Could you check a few things on this model? Use its own coordinates, in mm. Give positions to 0.01 mm unless a question says otherwise; leave off trailing zeros. Write each loop counter-clockwise with the first axis right and the second up, starting at its lowest first coordinate (ties: lowest second). Pieces come first, ordered by that corner, then holes. Notation, with made-up numbers: (58.25, -6) - (84.25, -6) arc R30 cw to (84.25, 31) - close; hole circle Ø2 at (58, 40). An arc over 180 degrees is marked (long way). Answer in a Markdown table with one row per item.
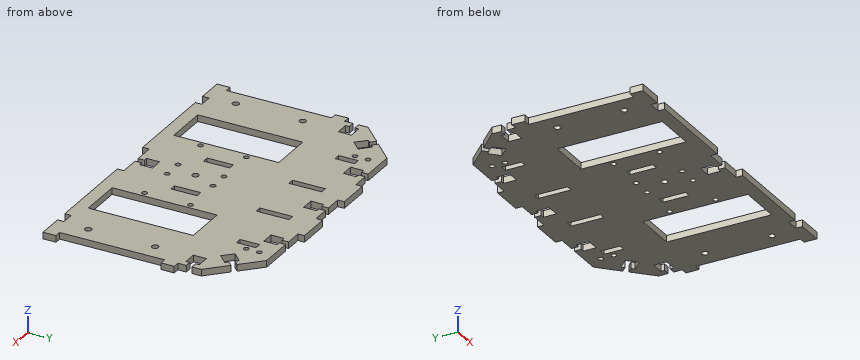
from build123d import *

# Parameters (mm, degrees)
BOSS_EXTRUDE1_DEPTH  = 5
BOSS_EXTRUDE2_DEPTH  = 5
SKETCH3_R            = 2
SKETCH3_R_2          = 2.5
CUT_EXTRUDE4_DEPTH   = 10
SKETCH6_R            = 2.5
CUT_EXTRUDE5_DEPTH   = 10
CUT_EXTRUDE6_DEPTH   = 10
SKETCH9_W            = 35
SKETCH9_H            = 5
SKETCH9_W_2          = 4.2
SKETCH9_W_3          = 10
SKETCH9_H_2          = 10
CUT_EXTRUDE7_DEPTH   = 10
SKETCH10_W           = 30.598870639
SKETCH10_H           = 58.148019952
CUT_EXTRUDE8_DEPTH   = 5
SKETCH11_W           = 30
SKETCH11_H           = 5
CUT_EXTRUDE9_DEPTH   = 5
SKETCH12_W           = 5
SKETCH12_H           = 80
BOSS_EXTRUDE3_DEPTH  = 4.5
SKETCH13_W           = 5
SKETCH13_H           = 80
BOSS_EXTRUDE4_DEPTH  = 4.5
SKETCH14_W           = 5
SKETCH14_H           = 5
BOSS_EXTRUDE5_DEPTH  = 0.1
SKETCH15_W           = 5
SKETCH15_H           = 5
CUT_EXTRUDE10_DEPTH  = 0.1
SKETCH16_W           = 5
SKETCH16_H           = 5
BOSS_EXTRUDE6_DEPTH  = 0.1
SKETCH17_W           = 5
SKETCH17_H           = 5
CUT_EXTRUDE11_DEPTH  = 0.1
SKETCH18_W           = 315.275634843
SKETCH18_H           = 155.272188677
CUT_EXTRUDE12_DEPTH  = 0.1
SKETCH19_W           = 15.4
SKETCH19_H           = 5
CUT_EXTRUDE13_DEPTH  = 0.1
CUT_EXTRUDE14_DEPTH  = 5
SKETCH21_W           = 5
SKETCH21_H           = 4.2
SKETCH21_W_2         = 3.2
SKETCH21_W_3         = 1.8
SKETCH21_H_2         = 1.4
CUT_EXTRUDE15_DEPTH  = 5
SKETCH22_W           = 5
SKETCH22_H           = 25
CUT_EXTRUDE16_DEPTH  = 10
SKETCH23_R           = 2
CUT_EXTRUDE17_DEPTH  = 10
CUT_EXTRUDE18_DEPTH  = 10
SKETCH25_W           = 5
SKETCH25_H           = 5
BOSS_EXTRUDE7_DEPTH  = 5
SKETCH28_W           = 10
SKETCH28_H           = 5
CUT_EXTRUDE19_DEPTH  = 5
SKETCH30_W           = 5
SKETCH30_H           = 15
CUT_EXTRUDE21_DEPTH  = 5
SKETCH31_W           = 10
SKETCH31_H           = 10
CUT_EXTRUDE22_DEPTH  = 10
SKETCH32_W           = 5
SKETCH32_H           = 10
CUT_EXTRUDE23_DEPTH  = 5
SKETCH33_W           = 5
SKETCH33_H           = 10
CUT_EXTRUDE24_DEPTH  = 5
SKETCH34_W           = 5
SKETCH34_H           = 80
BOSS_EXTRUDE10_DEPTH = 17.5
SKETCH35_W           = 5
SKETCH35_H           = 80
BOSS_EXTRUDE11_DEPTH = 17.5


with BuildPart() as part:
    # Sketch1 → Boss-Extrude1 (new body)
    with BuildSketch(Plane.XY):
        Polygon((-42.5, -104.9), (42.5, -104.9), (42.5, -49.9), (42.5, -37.4), (120, -37.4), (120, -17.4), (115, -17.4), (115, 12.8), (120, 12.8), (120, 27.7), (100.1, 27.7), (100.1, 22.7), (39.9, 22.7), (39.9, 27.7), (-39.9, 27.7), (-39.9, 22.7), (-100.1, 22.7), (-100.1, 27.7), (-120, 27.7), (-120, 12.8), (-115, 12.8), (-115, -17.4), (-120, -17.4), (-120, -37.4), (-42.5, -37.4), (-42.5, -49.9), align=None)
    extrude(amount=BOSS_EXTRUDE1_DEPTH)

    # Sketch2 → Boss-Extrude2 (add)
    with BuildSketch(Plane.XY.offset(5)):
        Polygon((-2.1, -104.9), (-42.5, -104.9), (-42.5, -117.4), (-93, -117.4), (-93, -37.4), (-110.5, -37.4), (-110.5, -117.4), (-120, -117.4), (-120, -127.4), (120, -127.4), (120, -117.4), (110.5, -117.4), (110.5, -37.4), (93, -37.4), (93, -117.4), (42.5, -117.4), (42.5, -104.9), (2.1, -104.9), align=None)
    extrude(amount=-BOSS_EXTRUDE2_DEPTH)

    # Sketch3 → Cut-Extrude4 (cut)
    with BuildSketch(Plane.XY.offset(5)):
        with Locations((-38.5, -59.9)):
            Circle(SKETCH3_R)
        with Locations((-38.5, -94.9)):
            Circle(SKETCH3_R)
        with Locations((-7.5, -94.9)):
            Circle(SKETCH3_R)
        with Locations((-7.5, -59.9)):
            Circle(SKETCH3_R)
        with Locations((38.5, -94.9)):
            Circle(SKETCH3_R)
        with Locations((7.5, -94.9)):
            Circle(SKETCH3_R)
        with Locations((7.5, -59.9)):
            Circle(SKETCH3_R)
        with Locations((38.5, -59.9)):
            Circle(SKETCH3_R)
        with Locations((0, -77.4)):
            Circle(SKETCH3_R_2)
    extrude(amount=-CUT_EXTRUDE4_DEPTH, mode=Mode.SUBTRACT)

    # Sketch6 → Cut-Extrude5 (cut)
    with BuildSketch(Plane.XY.offset(5)):
        with Locations((-101.75, -51.9)):
            Circle(SKETCH6_R)
        with Locations((-101.75, -102.9)):
            Circle(SKETCH6_R)
        with Locations((101.75, -102.9)):
            Circle(SKETCH6_R)
        with Locations((101.75, -51.9)):
            Circle(SKETCH6_R)
    extrude(amount=-CUT_EXTRUDE5_DEPTH, mode=Mode.SUBTRACT)

    # Sketch8 → Cut-Extrude6 (cut)
    with BuildSketch(Plane.XY.offset(5)):
        Polygon((-115, 22.7), (-90, 22.7), (-115, -2.3), align=None)
        Polygon((-115, 22.7), (-100.1, 22.7), (-100.1, 27.7), (-120, 27.7), (-120, 12.8), (-115, 12.8), align=None)
        Polygon((100.1, 22.7), (115, 22.7), (115, 12.8), (120, 12.8), (120, 27.7), (100.1, 27.7), align=None)
        Polygon((115, 12.8), (115, 22.7), (100.1, 22.7), (90, 22.7), (115, -2.3), align=None)
    extrude(amount=-CUT_EXTRUDE6_DEPTH, mode=Mode.SUBTRACT)

    # Sketch9 → Cut-Extrude7 (cut)
    with BuildSketch(Plane.XY.offset(5)):
        with Locations((0, -124.9)):
            Rectangle(SKETCH9_W, SKETCH9_H)
        with Locations((0, -119.9)):
            Rectangle(SKETCH9_W_2, SKETCH9_H)
        with Locations((0, -112.4)):
            Rectangle(SKETCH9_W_3, SKETCH9_H_2)
    extrude(amount=-CUT_EXTRUDE7_DEPTH, mode=Mode.SUBTRACT)

    # Sketch10 → Cut-Extrude8 (cut)
    with BuildSketch(Plane(origin=(-56.35, 56.35, 0), x_dir=(0, 0, 1), z_dir=(-0.707106781, 0.707106781, 0))):
        with Locations((4.930158629, -62.874909177)):
            Rectangle(SKETCH10_W, SKETCH10_H)
    cut_extrude8 = extrude(amount=-CUT_EXTRUDE8_DEPTH, mode=Mode.SUBTRACT)

    # Mirror1: Cut-Extrude8 across plane
    add(cut_extrude8.mirror(Plane(origin=(0, 0, 0), x_dir=(0, 0, 1), z_dir=(1, 0, 0))), mode=Mode.SUBTRACT)

    # Sketch11 → Cut-Extrude9 (cut)
    with BuildSketch(Plane.XY.offset(5)):
        with Locations((0, 25.2)):
            Rectangle(SKETCH11_W, SKETCH11_H)
    extrude(amount=-CUT_EXTRUDE9_DEPTH, mode=Mode.SUBTRACT)

    # Sketch12 → Boss-Extrude3 (add)
    with BuildSketch(Plane(origin=(110.5, 0, 0), x_dir=(0, 0, -1), z_dir=(1, 0, 0))):
        with Locations((-2.5, -77.4)):
            Rectangle(SKETCH12_W, SKETCH12_H)
    extrude(amount=BOSS_EXTRUDE3_DEPTH)

    # Sketch13 → Boss-Extrude4 (add)
    with BuildSketch(Plane.ZY.offset(110.5)):
        with Locations((2.5, -77.4)):
            Rectangle(SKETCH13_W, SKETCH13_H)
    extrude(amount=BOSS_EXTRUDE4_DEPTH)

    # Sketch14 → Boss-Extrude5 (add)
    with BuildSketch(Plane(origin=(0, -17.4, 0), x_dir=(1, 0, 0), z_dir=(0, 1, 0))):
        with Locations((117.5, -2.5)):
            Rectangle(SKETCH14_W, SKETCH14_H)
    extrude(amount=BOSS_EXTRUDE5_DEPTH)

    # Sketch15 → Cut-Extrude10 (cut)
    with BuildSketch(Plane.XZ.offset(37.4)):
        with Locations((117.5, 2.5)):
            Rectangle(SKETCH15_W, SKETCH15_H)
    extrude(amount=-CUT_EXTRUDE10_DEPTH, mode=Mode.SUBTRACT)

    # Sketch16 → Boss-Extrude6 (add)
    with BuildSketch(Plane(origin=(0, -17.4, 0), x_dir=(1, 0, 0), z_dir=(0, 1, 0))):
        with Locations((-117.5, -2.5)):
            Rectangle(SKETCH16_W, SKETCH16_H)
    extrude(amount=BOSS_EXTRUDE6_DEPTH)

    # Sketch17 → Cut-Extrude11 (cut)
    with BuildSketch(Plane.XZ.offset(37.4)):
        with Locations((-117.5, 2.5)):
            Rectangle(SKETCH17_W, SKETCH17_H)
    extrude(amount=-CUT_EXTRUDE11_DEPTH, mode=Mode.SUBTRACT)

    # Sketch18 → Cut-Extrude12 (cut)
    with BuildSketch(Plane.XZ.offset(127.4)):
        with Locations((9.753929885, -1.918428582)):
            Rectangle(SKETCH18_W, SKETCH18_H)
    extrude(amount=-CUT_EXTRUDE12_DEPTH, mode=Mode.SUBTRACT)

    # Sketch19 → Cut-Extrude13 (cut)
    with BuildSketch(Plane.XZ.offset(122.4)):
        with Locations((9.8, 2.5)):
            Rectangle(SKETCH19_W, SKETCH19_H)
        with Locations((-9.8, 2.5)):
            Rectangle(SKETCH19_W, SKETCH19_H)
    extrude(amount=-CUT_EXTRUDE13_DEPTH, mode=Mode.SUBTRACT)

    # Sketch20 → Cut-Extrude14 (cut)
    with BuildSketch(Plane.XY.offset(5)):
        Polygon((-97.479541854, 8.149390335), (-100.449390335, 5.179541854), (-96.913856429, 1.644007948), (-93.944007948, 4.613856429), align=None)
        Polygon((-91.893398282, 6.664466094), (-98.964466094, -0.406601718), (-91.893398282, -7.47766953), (-84.82233047, -0.406601718), align=None)
    cut_extrude14 = extrude(amount=-CUT_EXTRUDE14_DEPTH, mode=Mode.SUBTRACT)

    # Mirror2: Cut-Extrude14 across plane
    add(cut_extrude14.mirror(Plane(origin=(0, 0, 0), x_dir=(0, 0, 1), z_dir=(1, 0, 0))), mode=Mode.SUBTRACT)

    # Sketch21 → Cut-Extrude15 (cut)
    with BuildSketch(Plane.XY.offset(5)):
        with Locations((-112.5, -18.8)):
            Rectangle(SKETCH21_W, SKETCH21_H)
        with Locations((-108.4, -18.8)):
            Rectangle(SKETCH21_W_2, SKETCH21_H)
        with Locations((-105.9, -18.8)):
            Rectangle(SKETCH21_W_3, SKETCH21_H)
        with Locations((-108.4, -16)):
            Rectangle(SKETCH21_W_2, SKETCH21_H_2)
        with Locations((-108.4, -21.6)):
            Rectangle(SKETCH21_W_2, SKETCH21_H_2)
    cut_extrude15 = extrude(amount=-CUT_EXTRUDE15_DEPTH, mode=Mode.SUBTRACT)

    # Sketch22 → Cut-Extrude16 (cut)
    with BuildSketch(Plane.XY.offset(5)):
        with Locations((22.5, -69.8)):
            Rectangle(SKETCH22_W, SKETCH22_H)
        with Locations((22.5, -4.8)):
            Rectangle(SKETCH22_W, SKETCH22_H)
        with Locations((-22.5, -4.8)):
            Rectangle(SKETCH22_W, SKETCH22_H)
        with Locations((-22.5, -69.8)):
            Rectangle(SKETCH22_W, SKETCH22_H)
    extrude(amount=-CUT_EXTRUDE16_DEPTH, mode=Mode.SUBTRACT)

    # Sketch23 → Cut-Extrude17 (cut)
    with BuildSketch(Plane.XY.offset(5)):
        with Locations((75, 12.7)):
            Circle(SKETCH23_R)
        with Locations((75, 2.7)):
            Circle(SKETCH23_R)
        with Locations((-75, 2.7)):
            Circle(SKETCH23_R)
        with Locations((-75, 12.7)):
            Circle(SKETCH23_R)
    extrude(amount=-CUT_EXTRUDE17_DEPTH, mode=Mode.SUBTRACT)

    # Mirror3: Cut-Extrude15 across plane
    add(cut_extrude15.mirror(Plane(origin=(0, 0, 0), x_dir=(0, 0, 1), z_dir=(1, 0, 0))), mode=Mode.SUBTRACT)

    # Sketch24 → Cut-Extrude18 (cut)
    with BuildSketch(Plane.XY.offset(5)):
        Polygon((-52.8, 17.7), (-52.8, 22.7), (-57, 22.7), (-57, 17.7), (-59.9, 17.7), (-59.9, 7.7), (-49.9, 7.7), (-49.9, 17.7), align=None)
        Polygon((59.9, 7.7), (59.9, 17.7), (57, 17.7), (57, 22.7), (52.8, 22.7), (52.8, 17.7), (49.9, 17.7), (49.9, 7.7), align=None)
        Polygon((2.1, 17.7), (2.1, 22.7), (-2.1, 22.7), (-2.1, 17.7), (-5, 17.7), (-5, 7.7), (5, 7.7), (5, 17.7), align=None)
    extrude(amount=-CUT_EXTRUDE18_DEPTH, mode=Mode.SUBTRACT)

    # Sketch25 → Boss-Extrude7 (add)
    with BuildSketch(Plane.XY.offset(5)):
        with Locations((-22.5, -59.8)):
            Rectangle(SKETCH25_W, SKETCH25_H)
        with Locations((22.5, -59.8)):
            Rectangle(SKETCH25_W, SKETCH25_H)
    extrude(amount=-BOSS_EXTRUDE7_DEPTH)

    # Sketch28 → Cut-Extrude19 (cut)
    with BuildSketch(Plane.XY.offset(5)):
        with Locations((-95, -124.8)):
            Rectangle(SKETCH28_W, SKETCH28_H)
        with Locations((95, -124.8)):
            Rectangle(SKETCH28_W, SKETCH28_H)
    extrude(amount=-CUT_EXTRUDE19_DEPTH, mode=Mode.SUBTRACT)

    # Sketch30 → Cut-Extrude21 (cut)
    with BuildSketch(Plane.XY.offset(5)):
        with Locations((-68, 0.2)):
            Rectangle(SKETCH30_W, SKETCH30_H)
        with Locations((68, 0.2)):
            Rectangle(SKETCH30_W, SKETCH30_H)
    extrude(amount=-CUT_EXTRUDE21_DEPTH, mode=Mode.SUBTRACT)

    # Sketch31 → Cut-Extrude22 (cut)
    with BuildSketch(Plane.XY.offset(5)):
        with Locations((105, -18.8)):
            Rectangle(SKETCH31_W, SKETCH31_H)
        with Locations((-105, -18.8)):
            Rectangle(SKETCH31_W, SKETCH31_H)
    extrude(amount=-CUT_EXTRUDE22_DEPTH, mode=Mode.SUBTRACT)

    # Sketch32 → Cut-Extrude23 (cut)
    with BuildSketch(Plane.XY.offset(5)):
        with Locations((-117.5, -22.3)):
            Rectangle(SKETCH32_W, SKETCH32_H)
    extrude(amount=-CUT_EXTRUDE23_DEPTH, mode=Mode.SUBTRACT)

    # Sketch33 → Cut-Extrude24 (cut)
    with BuildSketch(Plane.XY.offset(5)):
        with Locations((117.5, -22.3)):
            Rectangle(SKETCH33_W, SKETCH33_H)
    extrude(amount=-CUT_EXTRUDE24_DEPTH, mode=Mode.SUBTRACT)

    # Sketch34 → Boss-Extrude10 (add)
    with BuildSketch(Plane.ZY.offset(-93)):
        with Locations((2.5, -77.4)):
            Rectangle(SKETCH34_W, SKETCH34_H)
    extrude(amount=BOSS_EXTRUDE10_DEPTH)

    # Sketch35 → Boss-Extrude11 (add)
    with BuildSketch(Plane(origin=(-93, 0, 0), x_dir=(0, 0, -1), z_dir=(1, 0, 0))):
        with Locations((-2.5, -77.4)):
            Rectangle(SKETCH35_W, SKETCH35_H)
    extrude(amount=BOSS_EXTRUDE11_DEPTH)


solid = part.part
1) Will these pins go through, and if not, where does the flat tip stop? P1, Ø1, axis at y = 11, z = 4, coming from the -X side; P2, Ø3, axis at x = 101.75, y = -102.9, coming from the +Z side; P3, Ø1, axis at x = -9.5, z = 3, coming from the -Y side; P4, Ø2.5, axis at y = -82.5, z = 2.5, coming from the -X side.
Check values:
| item | result |
|---|---|
| P1 | stops at x = -95.13 |
| P2 | passes through |
| P3 | stops at y = -122.3 |
| P4 | stops at x = -115 |
2) Imagine slicing it at B-B (z = 3.75). State how many separate pieces and enclosed holes the cut face has, then the cut area to 3 significant figures.
Check values:
| item | result |
|---|---|
| separate pieces | 1 |
| enclosed holes | 25 |
| area | 26,500 mm2 |
3) Imagine slicing it at A-A (y = -51.9). List the corners of the cut face in (x, z) for me.
Check values:
| item | result |
|---|---|
| outline | (-115, 0) - (-104.25, 0) - (-104.25, 5) - (-115, 5) - close; (-99.25, 0) - (-75.5, 0) - (-75.5, 5) - (-99.25, 5) - close; (-42.5, 0) - (42.5, 0) - (42.5, 5) - (-42.5, 5) - close; (75.5, 0) - (99.25, 0) - (99.25, 5) - (75.5, 5) - close; (104.25, 0) - (115, 0) - (115, 5) - (104.25, 5) - close |
4) If I drill on line 1 (X direction, y = -16, z = 1.8); line 2 (Y direction, x = -38.5, z = 3.2); line 3 (X direction, y = -73, z = 1.7), over which ranges is the centre line in solid material (lowest first)?
Check values:
| item | result |
|---|---|
| line 1 | x = -115 to -110, -100 to -25, -20 to 20, 25 to 100, 110 to 115 |
| line 2 | y = -127.3 to -96.9, -92.9 to -61.9, -57.9 to 27.7 |
| line 3 | x = -115 to -75.5, -42.5 to -25, -20 to 20, 25 to 42.5, 75.5 to 115 |
